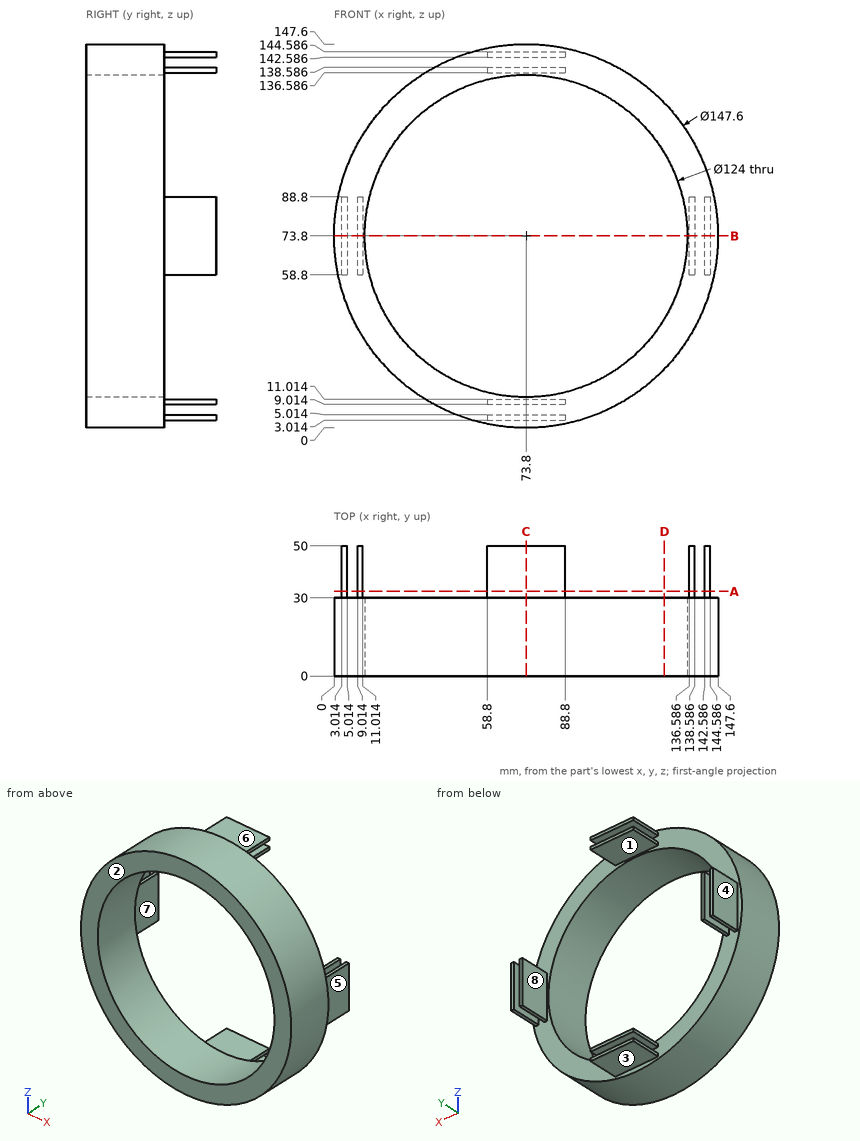
Verification items for this drawing (mm, ordinates from the low corner). A direction names the side the tool comes from. Coordinates: 2 decimals unless noted, no trailing zeros. Loops run counter-clockwise (first coordinate to the right, second up) from the corner with the lowest first, then second, coordinate; pieces in that order, holes last. Notation, with made-up numbers: (22, 18) - (61, 18) arc R15 ccw to (61, 39) - close; hole circle Ø5 at (83.5, -25). An arc over 180 degrees is marked (long way). Use one line per item in the form item = value. Start each with the question number.
Item 1: Thickness scan on probe 1 along Z at (x, y) = (84, 42); probe 2 along X at (y, z) = (22, 75.5). Record the ranges inside material, lowest first.
Item 2: Mould release check, pull along X, two halves, no side actions. Record for the marked faces 5, 6, 7 and 8: +X half, -X half, draft (parallel to the pull), parting line (faces both ways), or undercut.
Item 3: Section check D-D, the plane x = 127. Enter the section's corners in (y, z), and give its area (3 significant figures).
Item 4: Tool access check on the marked faces 1, 2, 3 and 4. Record the directions out of +Z, -Z, +X, -X, +Y, -Y that give a thin tool (end or side, any length) a straight path to the whole face; none if there is none.
Item 5: Section check A-A, the plane y = 32.5. Give the number of separate pieces and of enclosed holes in the cut face, and give its area (3 significant figures).
Item 6: Section check C-C, the plane x = 73.8. Enter the section's corners in (y, z).
Item 7: Gauge pin test, flat ends, axial feed: pin 1 (16 mm diameter, centred on x = 69.5, y = 42.5, fed in from +Z); pin 2 (10 mm diameter, centred on x = 29.5, y = 17.5, fed in from +Z) (1 decimal); pin 3 (5 mm diameter, centred on x = 83, y = 6, fed in from +Z) (1 decimal). Record the tip position at first contact, or that the pin passes through.
Item 8: Section check B-B, the plane z = 73.8. Enter the section's corners in (x, y), and give its area (3 significant figures).
Computed:
q1.probe_1 = 3.01 to 5.01, 9.01 to 11.01, 136.59 to 138.59, 142.59 to 144.59
q1.probe_2 = 0.02 to 11.82, 135.78 to 147.58
q2.face_5 = +X half
q2.face_6 = draft
q2.face_7 = undercut
q2.face_8 = undercut
q3.outline = (0, 22.65) - (30, 22.65) - (30, 41.96) - (0, 41.96) - close; (0, 105.64) - (30, 105.64) - (30, 124.95) - (0, 124.95) - close
q3.area = 1,160 mm2
q4.face_1 = +X, -X, +Y
q4.face_2 = +Z, -Z, +X, -X, -Y
q4.face_3 = -Z, +X, -X, +Y
q4.face_4 = +Z, -Z, -X, +Y
q5.separate_pieces = 8
q5.enclosed_holes = 0
q5.area = 480 mm2
q6.outline = (0, 0) - (30, 0) - (30, 3.01) - (50, 3.01) - (50, 5.01) - (30, 5.01) - (30, 9.01) - (50, 9.01) - (50, 11.01) - (30, 11.01) - (30, 11.8) - (0, 11.8) - close; (0, 135.8) - (30, 135.8) - (30, 136.59) - (50, 136.59) - (50, 138.59) - (30, 138.59) - (30, 142.59) - (50, 142.59) - (50, 144.59) - (30, 144.59) - (30, 147.6) - (0, 147.6) - close
q7.pin_1 = 144.59
q7.pin_2 = 136.3
q7.pin_3 = 147.3
q8.outline = (0, 0) - (11.8, 0) - (11.8, 30) - (11.01, 30) - (11.01, 50) - (9.01, 50) - (9.01, 30) - (5.01, 30) - (5.01, 50) - (3.01, 50) - (3.01, 30) - (0, 30) - close; (135.8, 0) - (147.6, 0) - (147.6, 30) - (144.59, 30) - (144.59, 50) - (142.59, 50) - (142.59, 30) - (138.59, 30) - (138.59, 50) - (136.59, 50) - (136.59, 30) - (135.8, 30) - close
q8.area = 868 mm2
